Build history of the part. All positions in model axes, mm. Give positions to 0.01 mm unless a question says otherwise; leave off trailing zeros. Order: outer loops, then holes, each group sorted by start corner. A loop starts at its lowest first (then second) coordinate and runs counter-clockwise, first axis right, second up. Notation, with made-up numbers: (-29.5, 13) - (15.5, 13) arc R21 ccw to (15.5, 27) - close; hole circle Ø8 at (-19.75, 66). An arc over 180 degrees is marked (long way). One line per item, written item: value.
```python
from build123d import *

# Parameters (mm, degrees)
SKETCH_W        = 50
SKETCH_H        = 40
PAD_DEPTH       = 20
SKETCH001_R     = 8.5
POCKET_DEPTH    = 40.001
SKETCH002_R     = 1.25
POCKET001_DEPTH = 20.001
FILLET_R        = 4


with BuildPart() as part:
    # Sketch → Pad (new body)
    with BuildSketch(Plane.XY):
        Rectangle(SKETCH_W, SKETCH_H)
    extrude(amount=PAD_DEPTH)

    # Sketch001 (on Face2 of Pad) → Pocket (cut, through all)
    with BuildSketch(Plane.XZ.offset(20)):
        Circle(SKETCH001_R)
    extrude(amount=-POCKET_DEPTH, mode=Mode.SUBTRACT)

    # Sketch002 (on Face5 of Pocket) → Pocket001 (cut, through all)
    with BuildSketch(Plane.XY.offset(20)):
        with Locations((-22, 17)):
            Circle(SKETCH002_R)
        with Locations((22, 17)):
            Circle(SKETCH002_R)
        with Locations((22, -17)):
            Circle(SKETCH002_R)
        with Locations((-22, -17)):
            Circle(SKETCH002_R)
    extrude(amount=-POCKET001_DEPTH, mode=Mode.SUBTRACT)

    # Fillet
    fillet_edges = [part.edges().sort_by_distance(p)[0] for p in [
        (-25, -20, 10),
        (-25, 20, 10),
        (25, 20, 10),
        (25, -20, 10),
    ]]
    fillet(fillet_edges, radius=FILLET_R)


solid = part.part
```
(1) Pull direction X, two halves, no side cores. Call faces 1 (the face through (23.19, 17.38, 10.14)), 2 (the face through (23.797, 18.859, 10.14)), 3 (the face through (-20.81, 17.38, 10.14)), 4 (the face through (-23.859, -18.797, 10.14)): +X half, -X half, draft (parallel to the pull), parting line (faces both ways), or undercut.
Completed:
face 1: undercut
face 2: +X half
face 3: undercut
face 4: -X half
(2) Drill centre lines: line 1 (Y direction, x = 22, z = 10.75); line 2 (Y direction, x = -23, z = 5.5); line 3 (X direction, y = -13, z = 2.5). Where is each one in solid material? Low to high.
Completed:
line 1: -19.87 to -18.25, -15.75 to 15.75, 18.25 to 19.87
line 2: -19.46 to -17.75, -16.25 to 16.25, 17.75 to 19.46
line 3: -25 to -8.12, 8.12 to 25
(3) Slice it at C-C, the plane z = 10.5. Give the cut face in (x, y), and give its area (3 significant figures).
Completed:
outline: (-25, -16) arc R4 ccw to (-21, -20) - (21, -20) arc R4 ccw to (25, -16) - (25, 16) arc R4 ccw to (21, 20) - (-21, 20) arc R4 ccw to (-25, 16) - close; hole circle Ø2.5 at (-22, -17); hole circle Ø2.5 at (-22, 17); hole circle Ø2.5 at (22, -17); hole circle Ø2.5 at (22, 17)
area: 1,970 mm²
(4) Slice it at D-D, the plane x = -22. Give the cut face in (y, z), and give its area (3 significant figures).
Completed:
outline: (-19.87, 0) - (-18.25, 0) - (-18.25, 20) - (-19.87, 20) - close; (-15.75, 0) - (15.75, 0) - (15.75, 20) - (-15.75, 20) - close; (18.25, 0) - (19.87, 0) - (19.87, 20) - (18.25, 20) - close
area: 695 mm²
(5) Slice it at B-B, the plane y = -17. Give the cut face in (x, z).
Completed:
outline: (-24.87, 0) - (-23.25, 0) - (-23.25, 20) - (-24.87, 20) - close; (-20.75, 0) - (-8.5, 0) arc R8.5 cw to (8.5, 0) - (20.75, 0) - (20.75, 20) - (-20.75, 20) - close; (23.25, 0) - (24.87, 0) - (24.87, 20) - (23.25, 20) - close
(6) Slice it at A-A, the plane z = 7. Give the cut face in (x, y), and give its area (3 significant figures).
Completed:
outline: (-25, -16) arc R4 ccw to (-21, -20) - (-4.82, -20) - (-4.82, 20) - (-21, 20) arc R4 ccw to (-25, 16) - close; (4.82, -20) - (21, -20) arc R4 ccw to (25, -16) - (25, 16) arc R4 ccw to (21, 20) - (4.82, 20) - close; hole circle Ø2.5 at (-22, -17); hole circle Ø2.5 at (-22, 17); hole circle Ø2.5 at (22, -17); hole circle Ø2.5 at (22, 17)
area: 1,580 mm²
